from build123d import *

# Parameters (mm, degrees)
SKETCH1_W           = 40
SKETCH1_H           = 20
BOSS_EXTRUDE1_DEPTH = 400
CUT_EXTRUDE3_DEPTH  = 401
CUT_EXTRUDE4_DEPTH  = 401
SKETCH6_R           = 2.3
CUT_EXTRUDE5_DEPTH  = 401


with BuildPart() as part:
    # Sketch1 → Boss-Extrude1 (new body)
    with BuildSketch(Plane.XY):
        with Locations((20, 10)):
            Rectangle(SKETCH1_W, SKETCH1_H)
    extrude(amount=-BOSS_EXTRUDE1_DEPTH)

    # Sketch2 → Cut-Extrude3 (cut, through all)
    with BuildSketch(Plane.XY):
        Polygon((14.58, 20), (13.395, 18.815), (13.395, 18.2), (15.5, 18.2), (15.5, 16.772792206), (12.627207794, 13.9), (7.372792206, 13.9), (4.5, 16.772792206), (4.5, 18.2), (6.605, 18.2), (6.605, 18.815), (5.42, 20), align=None)
        Polygon((1.185, 13.395), (0, 14.58), (0, 5.42), (1.185, 6.605), (1.8, 6.605), (1.8, 4.5), (3.227207794, 4.5), (6.1, 7.372792206), (6.1, 12.627207794), (3.227207794, 15.5), (1.8, 15.5), (1.8, 13.395), align=None)
        Polygon((38.2, 13.395), (38.815, 13.395), (40, 14.58), (40, 5.42), (38.815, 6.605), (38.2, 6.605), (38.2, 4.5), (36.772792206, 4.5), (33.9, 7.372792206), (33.9, 12.627207794), (36.772792206, 15.5), (38.2, 15.5), align=None)
        Polygon((33.395, 18.815), (34.58, 20), (25.42, 20), (26.605, 18.815), (26.605, 18.2), (24.5, 18.2), (24.5, 16.772792206), (27.372792206, 13.9), (32.627207794, 13.9), (35.5, 16.772792206), (35.5, 18.2), (33.395, 18.2), align=None)
        Polygon((33.395, 1.8), (33.395, 1.185), (34.58, 0), (25.42, 0), (26.605, 1.185), (26.605, 1.8), (24.5, 1.8), (24.5, 3.227207794), (27.372792206, 6.1), (32.627207794, 6.1), (35.5, 3.227207794), (35.5, 1.8), align=None)
        Polygon((6.605, 1.185), (5.42, 0), (14.58, 0), (13.395, 1.185), (13.395, 1.8), (15.5, 1.8), (15.5, 3.227207794), (12.627207794, 6.1), (7.372792206, 6.1), (4.5, 3.227207794), (4.5, 1.8), (6.605, 1.8), align=None)
    extrude(amount=-CUT_EXTRUDE3_DEPTH, mode=Mode.SUBTRACT)

    # Sketch5 → Cut-Extrude4 (cut, through all)
    with BuildSketch(Plane.XY):
        Polygon((17.3, 1.8), (22.7, 1.8), (22.7, 3.972792206), (26.1, 7.372792206), (26.1, 12.627207794), (22.7, 16.027207794), (22.7, 18.2), (17.3, 18.2), (17.3, 16.027207794), (13.9, 12.627207794), (13.9, 7.372792206), (17.3, 3.972792206), align=None)
    extrude(amount=-CUT_EXTRUDE4_DEPTH, mode=Mode.SUBTRACT)

    # Sketch6 → Cut-Extrude5 (cut, through all)
    with BuildSketch(Plane.XY):
        with Locations((10, 10)):
            Circle(SKETCH6_R)
        with Locations((30, 10)):
            Circle(SKETCH6_R)
    extrude(amount=-CUT_EXTRUDE5_DEPTH, mode=Mode.SUBTRACT)


solid = part.part
Design review of the part built by this model. Coordinates are the model's own, in mm. Coordinates: 2 decimals unless noted, no trailing zeros. Use one line per item in the form item = value.
Q1. For probe 1 along X at (y, z) = (10.5, -67) (3 decimals); probe 2 along X at (y, z) = (18.5, -279.5) (3 decimals); probe 3 along Y at (x, z) = (3, -81.5), list the stretches that pass through material, from the lowest coordinate up.
Taken from the geometry:
probe_1 = 6.1 to 7.755, 12.245 to 13.9, 26.1 to 27.755, 32.245 to 33.9
probe_2 = 0 to 6.605, 13.395 to 26.605, 33.395 to 40
probe_3 = 0 to 4.5, 15.5 to 20
Q2. Insertion check: pin 1 Ø6 at (y, z) = (10.5, -255.5) entering from -X; pin 2 Ø1.5 at (x, z) = (13.5, -281.5) entering from -Y; pin 3 Ø4 at (y, z) = (11, -150) entering from +X. Each pin has a flat end and moves straight along its axis. Give the tip position at first contact, or say it passes through.
Taken from the geometry:
pin_1 = 1.08
pin_2 = 0.33
pin_3 = 34.27
Q3. Consider section A-A (z = -340). Count the separate pieces of the cut face and the enclosed holes in it, plus the area to 3 significant figures.
Taken from the geometry:
separate_pieces = 1
enclosed_holes = 3
area = 303 mm^2
